Source: CAD feature listing. Evaluate the final solid. Frame: model axes, mm. A direction names the side the tool comes from. Round coordinates to 2 decimals unless told otherwise and drop trailing zeros. Loops run counter-clockwise (first coordinate to the right, second up) from the corner with the lowest first, then second, coordinate; pieces in that order, holes last. Notation, with made-up numbers: (-36, 45.5) - (-14, 45.5) arc R22 ccw to (-14, 75.5) - close; hole circle Ø2 at (85.25, 40). An arc over 180 degrees is marked (long way). Use CSV: the item, a comma, the result in double quotes. Start each with the question number.
from build123d import *

# Parameters (mm, degrees)
SKETCH1_R           = 64
BOSS_EXTRUDE2_DEPTH = 7
SKETCH3_R           = 37.5
SKETCH3_R_2         = 32.5
BOSS_EXTRUDE3_DEPTH = 12
SKETCH6_R           = 12.5
CUT_EXTRUDE1_DEPTH  = 8
FILLET1_R           = 2


with BuildPart() as part:
    # Sketch1 → Boss-Extrude2 (new body)
    with BuildSketch(Plane.XY):
        Circle(SKETCH1_R)
    extrude(amount=BOSS_EXTRUDE2_DEPTH)

    # Sketch3 → Boss-Extrude3 (add)
    with BuildSketch(Plane.XY.offset(7)):
        Circle(SKETCH3_R)
        Circle(SKETCH3_R_2, mode=Mode.SUBTRACT)
    extrude(amount=BOSS_EXTRUDE3_DEPTH)

    # Sketch6 → Cut-Extrude1 (cut, through all)
    with BuildSketch(Plane.XY.offset(7)):
        Circle(SKETCH6_R)
    extrude(amount=-CUT_EXTRUDE1_DEPTH, mode=Mode.SUBTRACT)

    # Fillet1
    fillet1_edges = [part.edges().sort_by_distance(p)[0] for p in [
        (-64, 0, 0),
        (-64, 0, 7),
        (-37.5, 0, 19),
    ]]
    fillet(fillet1_edges, radius=FILLET1_R)


solid = part.part
1. Reachability of faces 1 (the flat face through (16, -29, 19)), 2 (the flat face through (27, -27, 7)) from +Z, -Z, +X, -X, +Y, -Y: full face, straight path, thin tool, end or side. Return the list, or none.
2. Line query: line 1 along Y through (x, z) = (0, 13.5); line 2 along Y through (x, z) = (0, 2.5); line 3 along Z through (x, y) = (-16, -34.5). Output: solid intervals per line, ascending.
3. Contact query for flat-ended pins moving along their axis: P1, Ø4, axis at x = 28, y = 1.5, coming from the +Z side; P2, Ø8, axis at x = 26, z = 3, coming from the +Y side; P3, Ø10, axis at y = -6.5, z = 5.5, coming from the -X side. Output: stop coordinate, or through.
4. Section query C-C on z = 12. Return the cut outline in (x, y).
5. Section query A-A on y = 0. Return the cut outline in (x, z).
6. Mould query, pull axis X, two halves, no side actions, for faces 3 (the flat face through (13, 1, 0)), 4 (the cylindrical face through (-4.88, 37.18, 11.93)), 5 (the cylindrical face through (31, 9.76, 12.92)). Classes: +X half, -X half, draft (parallel to the pull), parting line (faces both ways), or undercut.
Values:
1,face 1,"+Z, +X, -X, +Y, -Y"
1,face 2,"+Z"
2,line 1,"y = -37.5 to -32.5, 32.5 to 37.5"
2,line 2,"y = -64 to -12.5, 12.5 to 64"
2,line 3,"z = 0 to 7"
3,P1,"stops at z = 7"
3,P2,"stops at y = 60.1"
3,P3,"stops at x = -63.98"
4,outline,"circle Ø75 at (0, 0); hole circle Ø65 at (0, 0)"
5,outline,"(-64, 2) arc R2 ccw to (-62, 0) - (-12.5, 0) - (-12.5, 7) - (-32.5, 7) - (-32.5, 19) - (-35.5, 19) arc R2 ccw to (-37.5, 17) - (-37.5, 7) - (-62, 7) arc R2 ccw to (-64, 5) - close; (12.5, 0) - (62, 0) arc R2 ccw to (64, 2) - (64, 5) arc R2 ccw to (62, 7) - (37.5, 7) - (37.5, 17) arc R2 ccw to (35.5, 19) - (32.5, 19) - (32.5, 7) - (12.5, 7) - close"
6,face 3,"draft"
6,face 4,"parting line"
6,face 5,"undercut"
